Could you check a few things on this model? Use its own coordinates, in mm. Give positions to 0.01 mm unless a question says otherwise; leave off trailing zeros. Loops run counter-clockwise (first coordinate to the right, second up) from the corner with the lowest first, then second, coordinate; pieces in that order, holes last. Notation, with made-up numbers: (28.5, -9) -> (62.5, -9) arc R24 ccw to (62.5, 3) -> close; hole circle Ø10 at (65.25, 56.25). An arc over 180 degrees is marked (long way). Put each result on its own line as item: value.
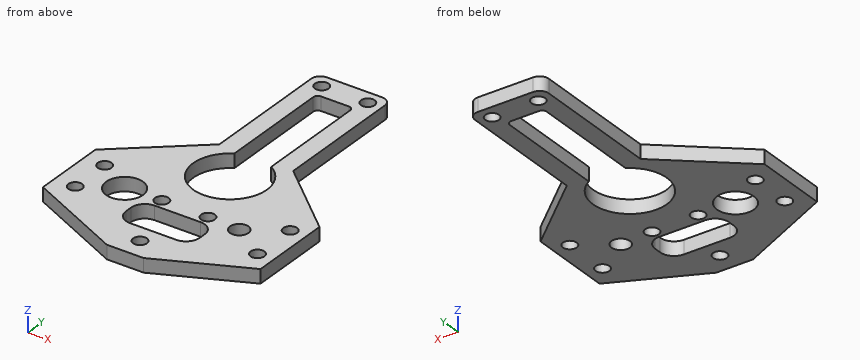
```python
from build123d import *

# Parameters (mm, degrees)
SKETCH1_R           = 1.5
SKETCH1_R_2         = 4
SKETCH1_R_3         = 2
BOSS_EXTRUDE1_DEPTH = 3


with BuildPart() as part:
    # Sketch1 → Boss-Extrude1 (new body)
    with BuildSketch(Plane.XY):
        with BuildLine():
            Line((-6, 70), (6, 70))
            ThreePointArc((6, 70), (7.414213562, 69.414213562), (8, 68))
            Line((8, 68), (8, 40))
            Line((8, 40), (23.052765378, 26.831315386))
            Line((23.052765378, 26.831315386), (23.052765378, 8.831315386))
            Line((23.052765378, 8.831315386), (4, 0))
            Line((4, 0), (-4, 0))
            Line((-4, 0), (-24.806216128, 9.803130645))
            Line((-24.806216128, 9.803130645), (-24.806216128, 25.803130645))
            Line((-24.806216128, 25.803130645), (-8, 40))
            Line((-8, 40), (-8, 68))
            ThreePointArc((-8, 68), (-7.414213562, 69.414213562), (-6, 70))
        make_face()
        with Locations((0, 4.5)):
            Circle(SKETCH1_R, mode=Mode.SUBTRACT)
        with Locations((-20.306216128, 13.303130645)):
            Circle(SKETCH1_R, mode=Mode.SUBTRACT)
        with Locations(Location((-20.311519457, 22.308427732, 0), (0, 0, 180))):
            Circle(SKETCH1_R, mode=Mode.SUBTRACT)
        with Locations((-12.806216128, 17.810197592)):
            Circle(SKETCH1_R_2, mode=Mode.SUBTRACT)
        with Locations((-5, 67)):
            Circle(SKETCH1_R, mode=Mode.SUBTRACT)
        with Locations(Location((5, 67, 0), (0, 0, 180))):
            Circle(SKETCH1_R, mode=Mode.SUBTRACT)
        with Locations((5, 18.2)):
            Circle(SKETCH1_R, mode=Mode.SUBTRACT)
        with Locations(Location((-5, 18.2, 0), (0, 0, 180))):
            Circle(SKETCH1_R, mode=Mode.SUBTRACT)
        with Locations((19.552765378, 12.829253326)):
            Circle(SKETCH1_R, mode=Mode.SUBTRACT)
        with Locations(Location((19.546876257, 22.829251592, 0), (0, 0, 180))):
            Circle(SKETCH1_R, mode=Mode.SUBTRACT)
        with Locations((12.052765378, 17.824837351)):
            Circle(SKETCH1_R_3, mode=Mode.SUBTRACT)
        with BuildLine():
            Line((-3, 64), (3, 64))
            ThreePointArc((3, 64), (3.707106781, 63.707106781), (4, 63))
            Line((4, 63), (4, 38.92820323))
            ThreePointArc((4, 38.92820323), (0, 24), (-4, 38.92820323))
            Line((-4, 38.92820323), (-4, 63))
            ThreePointArc((-4, 63), (-3.707106781, 63.707106781), (-3, 64))
        make_face(mode=Mode.SUBTRACT)
        with BuildLine():
            Line((-5, 16), (5, 16))
            ThreePointArc((5, 16), (7.121320344, 15.121320344), (8, 13))
            Line((8, 13), (8, 11.5))
            ThreePointArc((8, 11.5), (7.121320344, 9.378679656), (5, 8.5))
            Line((5, 8.5), (-5, 8.5))
            ThreePointArc((-5, 8.5), (-7.121320344, 9.378679656), (-8, 11.5))
            Line((-8, 11.5), (-8, 13))
            ThreePointArc((-8, 13), (-7.121320344, 15.121320344), (-5, 16))
        make_face(mode=Mode.SUBTRACT)
    extrude(amount=BOSS_EXTRUDE1_DEPTH)


solid = part.part
```
1. If we section it at A-A (y = 51): List the corners of the cut face in (x, z) for me, then the cut area to 3 significant figures.
Recorded:
outline: (-8, 0) -> (-4, 0) -> (-4, 3) -> (-8, 3) -> close; (4, 0) -> (8, 0) -> (8, 3) -> (4, 3) -> close
area: 24.0 mm^2
2. If we section it at C-C (z = 0.95): Count the separate pieces of the cut face and the enclosed holes in it, then the cut area to 3 significant figures.
Recorded:
separate pieces: 1
enclosed holes: 13
area: 1,350 mm^2
3. I need wall thicknesses on line 1 (Y direction, x = 0, z = 1.15); line 2 (X direction, y = 52, z = 1.4); line 3 (Y direction, x = 0.5, z = 1.85). Which ranges of each line are inside material? Lowest first, please.
Recorded:
line 1: y = 0 to 3, 6 to 8.5, 16 to 24, 64 to 70
line 2: x = -8 to -4, 4 to 8
line 3: y = 0 to 3.09, 5.91 to 8.5, 16 to 24.02, 64 to 70
4. If we section it at B-B (x = -10): List the corners of the cut face in (y, z) for me, then the cut area to 3 significant figures.
Recorded:
outline: (2.83, 0) -> (14.96, 0) -> (14.96, 3) -> (2.83, 3) -> close; (20.66, 0) -> (38.31, 0) -> (38.31, 3) -> (20.66, 3) -> close
area: 89.3 mm^2
5. If we section it at D-D (y = 7.5): List the corners of the cut face in (x, z) for me.
Recorded:
outline: (-19.92, 0) -> (20.18, 0) -> (20.18, 3) -> (-19.92, 3) -> close
6. I'm going to push flat-ended pins straight in: pin 1 (0.9 mm diameter, centred on y = 58.5, z = 1, fed in from +X); pin 2 (1.5 mm diameter, centred on y = 50.5, z = 2, fed in from -X). Where does each tip first touch, or does it pass through?
Recorded:
pin 1: stops at x = 8
pin 2: stops at x = -8
